from build123d import *

# Parameters (mm, degrees)
F1_DEPTH  = 53
F2_W      = 80
F2_H      = 25
F3_DEPTH  = 25
F4_W      = 23
F4_H      = 115.9437634051
F5_DEPTH  = 7
F6_W      = 34
F6_H      = 8.5
F7_DEPTH  = 50.001
F8_W      = 26
F8_H      = 4
F9_DEPTH  = 10
F10_R     = 2
F11_DEPTH = 10
F12_SIZE2 = 7
F12_SIZE  = 10
F13_SIZE2 = 10
F13_SIZE  = 7
F15_D     = 3.2
F15_DEPTH = 12
F15_TIP   = 0.9613769904
F16_R     = 3.99999


# Not quite as in the source:
# - a fillet or chamfer is up to 0.001 mm smaller than in the source, because OpenCascade refuses the exact size


with BuildPart() as f1:
    # F0 (on Right) → F1 (new body, symmetric)
    with BuildSketch(Plane.YZ):
        Polygon((44, 25), (-44, 25), (-44, -25), (-32.5, -25), (-32.5, -10), (-25, 3.5), (-6, 14.5), (0, 14.5), (6, 14.5), (25, 3.5), (32.5, -10), (32.5, -25), (44, -25), align=None)
    extrude(amount=F1_DEPTH, both=True)

    # F2 (on face) → F3 (cut)
    with BuildSketch(Plane.XY.offset(25)):
        Rectangle(F2_W, F2_H)
    extrude(amount=-F3_DEPTH, mode=Mode.SUBTRACT)

    # F4 (on face) → F5 (cut)
    with BuildSketch(Plane.XY.offset(25)):
        with Locations((-28.5, -2.7361307293)):
            Rectangle(F4_W, F4_H)
        with Locations((28.5, -2.7361307293)):
            Rectangle(F4_W, F4_H)
    extrude(amount=-F5_DEPTH, mode=Mode.SUBTRACT)

    # F6 (on face) → F7 (cut, through all)
    with BuildSketch(Plane.XY.offset(25)):
        with Locations((0, 16.75)):
            Rectangle(F6_W, F6_H)
        with Locations((0, -16.75)):
            Rectangle(F6_W, F6_H)
    extrude(amount=-F7_DEPTH, mode=Mode.SUBTRACT)

    # F8 (on face) → F9 (cut)
    with BuildSketch(Plane.XY.offset(25)):
        with Locations((0, 23)):
            Rectangle(F8_W, F8_H)
        with Locations((0, -23)):
            Rectangle(F8_W, F8_H)
    extrude(amount=-F9_DEPTH, mode=Mode.SUBTRACT)

    # F10 (on face) → F11 (cut)
    with BuildSketch(Plane.XY.offset(25)):
        with Locations((-13, 25)):
            Circle(F10_R)
        with Locations((13, 25)):
            Circle(F10_R)
        with Locations((-13, -25)):
            Circle(F10_R)
        with Locations((13, -25)):
            Circle(F10_R)
    extrude(amount=-F11_DEPTH, mode=Mode.SUBTRACT)

    # F12
    f12_edges = [f1.edges().sort_by_distance(p)[0] for p in [
        (-46.5, -44, 25),
        (0, -44, 25),
        (46.5, -44, 25),
    ]]
    chamfer(f12_edges, length=F12_SIZE, length2=F12_SIZE2)

    # F13
    f13_edges = [f1.edges().sort_by_distance(p)[0] for p in [
        (-46.5, 44, 25),
        (0, 44, 25),
        (46.5, 44, 25),
    ]]
    f13_side = f1.faces().sort_by_distance((0, 44, -1.390719))[0]
    chamfer(f13_edges, length=F13_SIZE, length2=F13_SIZE2, reference=f13_side)

    # F15
    with Locations(Plane.XY.offset(25)):
        with Locations((-47, 0), (47, 0)):
            Hole(F15_D / 2, depth=F15_DEPTH)
            with Locations((0, 0, -(F15_DEPTH + F15_TIP / 2))):  # 118° drill point
                Cone(0, F15_D / 2, F15_TIP, mode=Mode.SUBTRACT)

    # F16 (radius 4 in the source; OpenCascade refuses exactly that, so slightly less here)
    f16_edges = [f1.edges().sort_by_distance(p)[0] for p in [
        (17, 21, 11.907895),
        (-17, 21, 11.907895),
        (-40, 12.5, 14.368421),
        (-40, -12.5, 14.368421),
        (-17, -21, 11.907895),
        (17, -21, 11.907895),
        (40, -12.5, 14.368421),
        (40, 12.5, 14.368421),
    ]]
    fillet(f16_edges, radius=F16_R)


solid = f1.part
Geometry check sheet. Reference: the model listing, model coordinates, mm. A direction names the side the tool comes from. Give positions to 0.01 mm unless a question says otherwise; leave off trailing zeros. Loops run counter-clockwise (first coordinate to the right, second up) from the corner with the lowest first, then second, coordinate; pieces in that order, holes last.
(1) Release check for a two-part mould opening along X. For faces 1 (the flat face through (-53, -1, 17)), 2 (the flat face through (17, -15, 14)), 3 (the flat face through (1, 32.5, -17)), 4 (the flat face through (0, 25, 20)) record: released by +X, released by -X, zero draft, split by the parting line, or undercut.
From the geometry:
face 1: released by -X
face 2: undercut
face 3: zero draft
face 4: undercut
(2) Section check A-A on x = -28. Record the cut outline in (y, z), then the cut area to 3 significant figures.
From the geometry:
outline: (-44, -25) - (-32.5, -25) - (-32.5, -10) - (-25, 3.5) - (-12.5, 10.74) - (-12.5, 18) - (-44, 18) - close; (12.5, 10.74) - (25, 3.5) - (32.5, -10) - (32.5, -25) - (44, -25) - (44, 18) - (12.5, 18) - close
area: 1,580 mm2
(3) Set-up check for faces 5 (the flat face through (-17, 30, 22)), 6 (the cylindrical face through (14.367, -26.46, 20.07)), 7 (the flat face through (1, 38, -25)), 8 (the flat face through (0.74, 28.7, -3.16)), 9 (the cylindrical face through (15.797, 19.859, 11.823)): record each of +Z, -Z, +X, -X, +Y, -Y from which the full face is reachable in a straight line by a thin tool's end or side.
From the geometry:
face 5: +Z, +Y, -Y
face 6: +Z
face 7: -Z, +X, -X, +Y, -Y
face 8: -Z, +X, -X
face 9: +Z, -Z
(4) Section check C-C on y = 0. Record the cut outline in (x, z), then the cut area to 3 significant figures.
From the geometry:
outline: (-53, 14.5) - (-48.6, 14.5) - (-48.6, 25) - (-53, 25) - close; (-45.4, 14.5) - (-40, 14.5) - (-40, 25) - (-45.4, 25) - close; (40, 14.5) - (45.4, 14.5) - (45.4, 25) - (40, 25) - close; (48.6, 14.5) - (53, 14.5) - (53, 25) - (48.6, 25) - close
area: 206 mm2
(5) Section check D-D on y = -19.5. Record the cut outline in (x, z), then the cut area to 3 significant figures.
From the geometry:
outline: (-53, 6.68) - (-16.12, 6.68) - (-16.12, 18) - (-40, 18) - (-40, 25) - (-53, 25) - close; (16.12, 6.68) - (53, 6.68) - (53, 25) - (40, 25) - (40, 18) - (16.12, 18) - close
area: 1,020 mm2
(6) Depth check by flat-ended pin: pin 1 Ø6 at (x, y) = (-34, 21.5) entering from +Z; pin 2 Ø1.5 at (x, y) = (24.5, 23.5) entering from -Z. Enter the tip coordinate at first touch or a pass-through.
From the geometry:
pin 1: stops at z = 18
pin 2: stops at z = 3.93
(7) Section check B-B on z = 20. Count the separate pieces of the cut face and the enclosed holes in it, then the cut area to 3 significant figures.
From the geometry:
separate pieces: 4
enclosed holes: 2
area: 3,250 mm2
(8) Thickness scan on L1, parallel to X at y = 40, z = 18.5; L2, parallel to Y at x = 11, z = -16.5; L3, parallel to Y at x = -7, z = 9. Record the ranges inside material, lowest first.
From the geometry:
L1: x = -53 to -40, -17 to 17, 40 to 53
L2: y = -44 to -32.5, 32.5 to 44
L3: y = -44 to -21, 21 to 44
